Work out the finished part from the listing and answer in its coordinate system (mm). Face numbers are marked on the shaded views. A direction names the side the tool comes from. Coordinates: 2 decimals unless noted, no trailing zeros. Write each loop counter-clockwise with the first axis right and the second up, starting at its lowest first coordinate (ties: lowest second). Pieces come first, ordered by that corner, then holes. Notation, with made-up numbers: (74.25, 17) - (112.25, 17) arc R25 cw to (112.25, 56) - close; hole circle Ø6 at (4, -30). An arc over 180 degrees is marked (long way). Use a Markdown table: item, result. Add a question column.
(1) Given pin 1 Ø12.5 at (y, z) = (-16.5, 25) entering from +X; pin 2 Ø3.5 at (x, z) = (-34, 30) entering from +Y; pin 3 Ø4 at (x, y) = (6.5, -6.5) entering from +Z, each flat-ended and moving along its own axis, determine where each tip first touches the part or whether it passes through.
(2) Find the intervals of material crossed by line 1 (X direction, y = -12, z = -4.5); line 2 (X direction, y = -14, z = -6); line 3 (X direction, y = -11.5, z = 14.5), in increasing order. Write a range as from..to.
(3) For a pull along Y with two mould halves and no side action, classify the marked faces 4, 5 and 6 as released by +Y, released by -Y, zero draft, split by the parting line, or undercut.
(4) A tool of negligible diameter and unlimited length cuts with its end or side. For the marked faces 1, 2 and 3, from which of +Z, -Z, +X, -X, +Y, -Y can it reach the whole face along a straight path? Write none if from no direction.
(5) The part is cut by section A-A, the plane z = 19.5. Give the vertices of the cut face in (x, y), then the cut area to 3 significant figures.
(6) The part is cut by section D-D, the plane x = -32.5. Give the vertices of the cut face in (y, z).
(7) The part is cut by section C-C, the plane y = -16. Give the vertices of the cut face in (x, z), then the cut area to 3 significant figures.
(8) The part is cut by section B-B, the plane x = 5.5. Give the vertices of the cut face in (y, z), then the cut area to 3 significant figures.
from build123d import *

# Parameters (mm, degrees)
F1_DEPTH = 25.4
F3_DEPTH = 25.4
F5_DEPTH = 25.4
F6_R     = 7.129897
F6_R_2   = 6.832178
F7_DEPTH = 25.4


with BuildPart() as f1:
    # F0 (on Front) → F1 (new body)
    with BuildSketch(Plane.XZ):
        Polygon((-25.733615, 35.668769), (-38.433615, 35.668769), (-38.433615, -8.781231), (25.066385, -8.781231), (25.066385, 3.918769), (-25.733615, 3.918769), align=None)
    extrude(amount=F1_DEPTH)

    # F2 (on face) → F3 (cut)
    with BuildSketch(Plane.YZ.offset(-25.733615)):
        with BuildLine():
            ThreePointArc((-25.4, 24.146574), (-11.982597, 34.99752), (0, 22.580311))
            Line((0, 22.580311), (0, 35.668769))
            Line((0, 35.668769), (-25.4, 35.668769))
            Line((-25.4, 35.668769), (-25.4, 24.146574))
        make_face()
    extrude(amount=-F3_DEPTH, mode=Mode.SUBTRACT)

    # F4 (on face) → F5 (cut)
    with BuildSketch(Plane.YZ.offset(-25.733615)):
        with BuildLine():
            ThreePointArc((-8.279151, 34.206712), (-13.009328, 35.01947), (-17.705537, 34.029128))
            Line((-17.705537, 34.029128), (-17.705537, 21.797176))
            ThreePointArc((-17.705537, 21.797176), (-13.126532, 16.82113), (-8.279151, 21.53613))
            Line((-8.279151, 21.53613), (-8.279151, 34.206712))
        make_face()
    extrude(amount=-F5_DEPTH, mode=Mode.SUBTRACT)

    # F6 (on face) → F7 (cut)
    with BuildSketch(Plane.XY.offset(3.918769)):
        with Locations((-15.662644, -11.877504)):
            Circle(F6_R)
        with Locations((6.787145, -13.182725)):
            Circle(F6_R_2)
        with BuildLine():
            ThreePointArc((13.574292, 0), (24.730975, -11.963104), (15.401599, -25.4))
            Line((15.401599, -25.4), (25.066385, -25.4))
            Line((25.066385, -25.4), (25.066385, 0))
            Line((25.066385, 0), (13.574292, 0))
        make_face()
    extrude(amount=-F7_DEPTH, mode=Mode.SUBTRACT)


solid = f1.part
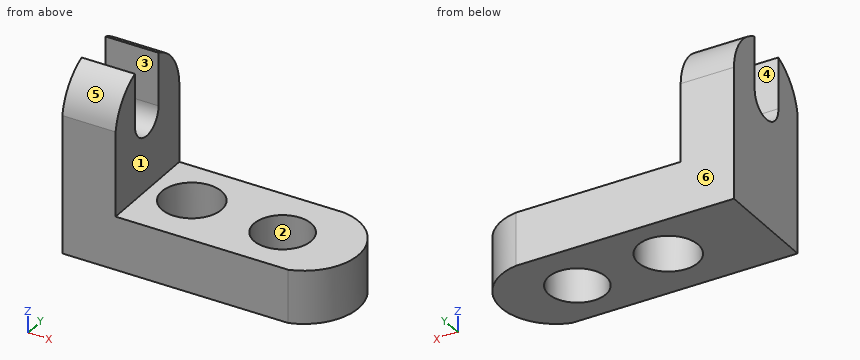
Model answer:
| question | item | result |
|---|---|---|
| 1 | pin 1 | x = -25.73 |
| 1 | pin 2 | y = -1.49 |
| 1 | pin 3 | z = 3.92 |
| 2 | line 1 | -38.43..-22.79, -8.53..0.06, 13.52..24.73 |
| 2 | line 2 | -38.43..-22.47, -8.86..0, 13.57..24.72 |
| 2 | line 3 | -38.43..-25.73 |
| 3 | face 4 | undercut |
| 3 | face 5 | released by -Y |
| 3 | face 6 | released by +Y |
| 4 | face 1 | +Z, +X, +Y, -Y |
| 4 | face 2 | +Z, -Z |
| 4 | face 3 | +Z, +X, -X |
| 5 | outline | (-38.43, -25.4) - (-25.73, -25.4) - (-25.73, -17.25) - (-38.43, -17.25) - close; (-38.43, -8.74) - (-25.73, -8.74) - (-25.73, 0) - (-38.43, 0) - close |
| 5 | area | 215 mm^2 |
| 6 | outline | (-25.4, -8.78) - (0, -8.78) - (0, 22.58) arc R12.77 ccw to (-8.28, 34.21) - (-8.28, 21.54) arc R4.72 cw (long way) to (-17.71, 21.8) - (-17.71, 34.03) arc R12.77 ccw to (-25.4, 24.15) - close |
| 7 | outline | (-38.43, -8.78) - (-21.48, -8.78) - (-21.48, 3.92) - (-25.73, 3.92) - (-25.73, 17.9) - (-38.43, 17.9) - close; (-9.85, -8.78) - (0.56, -8.78) - (0.56, 3.92) - (-9.85, 3.92) - close; (13.01, -8.78) - (24.39, -8.78) - (24.39, 3.92) - (13.01, 3.92) - close |
| 7 | area | 670 mm^2 |
| 8 | outline | (-25.4, -8.78) - (-19.89, -8.78) - (-19.89, 3.92) - (-25.4, 3.92) - close; (-6.47, -8.78) - (0, -8.78) - (0, 3.92) - (-6.47, 3.92) - close |
| 8 | area | 152 mm^2 |
